Drawing for the job (mm, zero at the part's lowest x, y, z). Give positions to 0.01 mm unless a question says otherwise; leave off trailing zeros. Order: outer loops, then holes, each group sorted by start corner. A loop starts at its lowest first (then second) coordinate and runs counter-clockwise, first axis right, second up. Notation, with made-up numbers: M -20.75,61 L 1.25,61 A23 cw 1.25,91 Z; hole C -4,6 d11. An arc over 180 degrees is marked long. Answer as a JSON object with one key per item and string values.
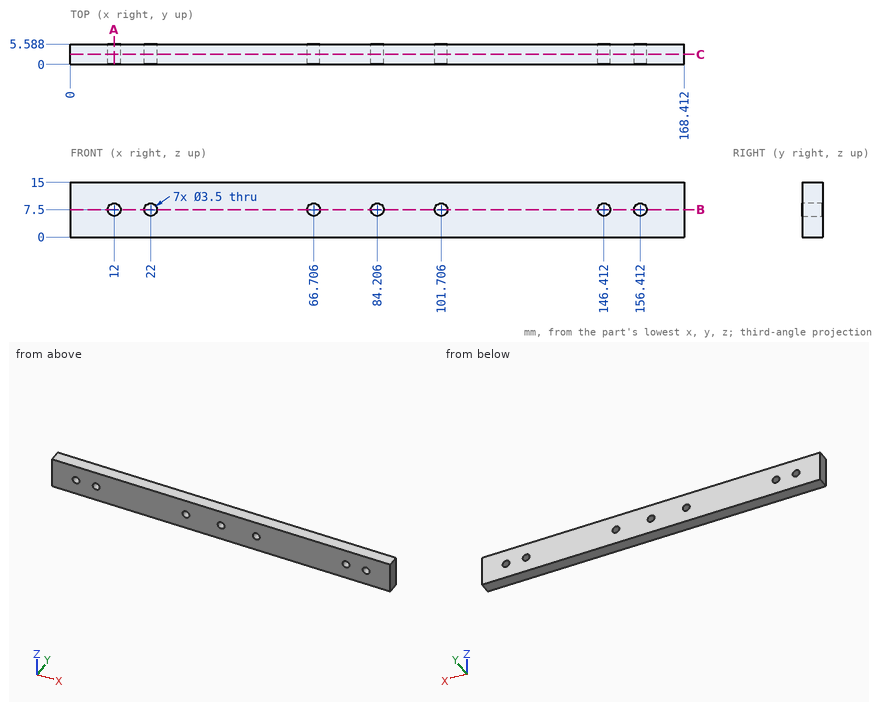
1. Pin check, flat tip, straight feed: P1, Ø4, axis at x = 146.412, z = 7.5, coming from the -Y side. Stop position of the tip, or through.
Worked answers:
{"P1": "stops at y = 0"}
2. Cut at A-A on x = 12. Give the cut face in (y, z), plus the area to 3 significant figures.
Worked answers:
{"outline": "M 0,0 L 5.59,0 L 5.59,5.75 L 0,5.75 Z; M 0,9.25 L 5.59,9.25 L 5.59,15 L 0,15 Z", "area": "64.3 mm^2"}
3. Cut at B-B on z = 7.5. State how many separate pieces and enclosed holes the cut face has, plus the area to 3 significant figures.
Worked answers:
{"separate pieces": "8", "enclosed holes": "0", "area": "804 mm^2"}
4. Cut at C-C on y = 2.75. Give the cut face in (x, z).
Worked answers:
{"outline": "M 0,0 L 168.41,0 L 168.41,15 L 0,15 Z; hole C 12,7.5 d3.5; hole C 22,7.5 d3.5; hole C 66.71,7.5 d3.5; hole C 84.21,7.5 d3.5; hole C 101.71,7.5 d3.5; hole C 146.41,7.5 d3.5; hole C 156.41,7.5 d3.5"}
